```python
from build123d import *

# Parameters (mm, degrees)
EXTRUDE003_DEPTH           = 10
EXTRUDE003_PLACEMENT_ANGLE = 90
SKETCH002_R                = 2.7
EXTRUDE002_DEPTH           = 25
SKETCH001_R                = 5.2
EXTRUDE001_DEPTH           = 6
SKETCH_R                   = 13
SKETCH_R_2                 = 1.65
EXTRUDE_DEPTH              = 5
BOX002_W                   = 43
BOX002_H                   = 42.3
BOX002_DEPTH               = 20
CHAMFER_SIZE               = 4
BOX001_W                   = 20.5
BOX001_H                   = 20.5
BOX001_DEPTH               = 25
BOX_W                      = 63.5
BOX_H                      = 71
BOX_DEPTH                  = 25
CHAMFER001_1_SIZE          = 15
CHAMFER001_2_SIZE          = 2
FILLET_R                   = 1


with BuildPart() as obj1:
    # Sketch003 → Extrude003 (new body)
    with BuildSketch(Plane.YZ):
        with BuildLine():
            ThreePointArc((-3.676943, 3.676968), (0, -5.2), (3.676943, 3.676968))
            Line((2.153911, 5.2), (3.676943, 3.676968))
            Line((-2.153911, 5.2), (2.153911, 5.2))
            Line((-3.676943, 3.676968), (-2.153911, 5.2))
        make_face()
    extrude(amount=EXTRUDE003_DEPTH)


with BuildPart() as obj1_1:
    # Extrude003 placement: moved
    add(obj1.part.moved(Location((42, 62, 10.2))).rotate(Axis((42, 62, 10.2), (0, 0, 1)), EXTRUDE003_PLACEMENT_ANGLE))


with BuildPart() as obj2:
    # Sketch002 → Extrude002 (new body)
    with BuildSketch(Plane.XY):
        with Locations((31.5, 10.25)):
            Circle(SKETCH002_R)
        with Locations((52.5, 10.25)):
            Circle(SKETCH002_R)
        with Locations((10.25, 32.5)):
            Circle(SKETCH002_R)
        with Locations((10.25, 58.8)):
            Circle(SKETCH002_R)
    extrude(amount=EXTRUDE002_DEPTH)


with BuildPart() as huecos:
    # Sketch001 → Extrude001 (new body)
    with BuildSketch(Plane.XY):
        with Locations((31.5, 10.25)):
            Circle(SKETCH001_R)
        with Locations((52.5, 10.25)):
            Circle(SKETCH001_R)
        with Locations((10.25, 32.5)):
            Circle(SKETCH001_R)
        with Locations((10.25, 58.8)):
            Circle(SKETCH001_R)
    extrude(amount=EXTRUDE001_DEPTH)

    # Fusion001: union obj2
    add(obj2.part)

    # Fusion002: union obj1
    add(obj1_1.part)


with BuildPart() as agujero_motor:
    # Sketch → Extrude (new body)
    with BuildSketch(Plane(origin=(20.5, 20.5, 25), x_dir=(1, 0, 0), z_dir=(0, 0, 1))):
        with Locations((21.5, 21.5)):
            Circle(SKETCH_R)
        with Locations((6, 37)):
            Circle(SKETCH_R_2)
        with Locations((37, 37)):
            Circle(SKETCH_R_2)
        with Locations((37, 6)):
            Circle(SKETCH_R_2)
        with Locations((6, 6)):
            Circle(SKETCH_R_2)
    extrude(amount=EXTRUDE_DEPTH)


with BuildPart() as agujero_motor_1:
    # Extrude placement: moved
    add(agujero_motor.part.moved(Location((0, 0, -25))))


with BuildPart() as hueco_motor_total:
    # Box002 → Box002 (new body)
    with BuildSketch(Plane(origin=(20.5, 20.5, 5), x_dir=(1, 0, 0), z_dir=(0, 0, 1))):
        with Locations((21.5, 21.15)):
            Rectangle(BOX002_W, BOX002_H)
    extrude(amount=BOX002_DEPTH)

    # Chamfer
    chamfer_edges = [hueco_motor_total.edges().sort_by_distance(p)[0] for p in [
        (20.5, 20.5, 15),
        (20.5, 62.8, 15),
    ]]
    chamfer(chamfer_edges, length=CHAMFER_SIZE)

    # Fusion: union agujero_motor
    add(agujero_motor_1.part)


with BuildPart() as obj3:
    # Box001 → Box001 (new body)
    with BuildSketch(Plane.XY):
        with Locations((10.25, 10.25)):
            Rectangle(BOX001_W, BOX001_H)
    extrude(amount=BOX001_DEPTH)


with BuildPart() as obj4:
    # Box → Box (new body)
    with BuildSketch(Plane.XY):
        with Locations((31.75, 35.5)):
            Rectangle(BOX_W, BOX_H)
    extrude(amount=BOX_DEPTH)

    # Cut: cut obj3
    add(obj3.part, mode=Mode.SUBTRACT)

    # Cut001: cut hueco_motor_total
    add(hueco_motor_total.part, mode=Mode.SUBTRACT)

    # Cut002: cut huecos
    add(huecos.part, mode=Mode.SUBTRACT)

    # Chamfer001 1
    chamfer001_1_edges = [obj4.edges().sort_by_distance(p)[0] for p in [
        (63.5, 66.9, 25),
    ]]
    chamfer(chamfer001_1_edges, length=CHAMFER001_1_SIZE)

    # Chamfer001 2
    chamfer001_2_edges = [obj4.edges().sort_by_distance(p)[0] for p in [
        (63.5, 10.25, 25),
    ]]
    chamfer(chamfer001_2_edges, length=CHAMFER001_2_SIZE)

    # Fillet
    fillet_edges = [obj4.edges().sort_by_distance(p)[0] for p in [
        (63.5, 71, 5),
        (0, 71, 12.5),
        (0, 20.5, 12.5),
        (20.5, 0, 12.5),
        (63.5, 0, 11.5),
    ]]
    fillet(fillet_edges, radius=FILLET_R)


solid = obj4.part
```
The listing builds one solid part. Answer for the finished solid, in the listing's coordinates (mm). A direction names the side the tool comes from. Give positions to 0.01 mm unless a question says otherwise; leave off trailing zeros. Order: outer loops, then holes, each group sorted by start corner. A loop starts at its lowest first (then second) coordinate and runs counter-clockwise, first axis right, second up. Notation, with made-up numbers: (39.5, -29) -> (60.5, -29) arc R25 ccw to (60.5, 1) -> close; hole circle Ø10 at (45, 89.5). An arc over 180 degrees is marked (long way). Write each question's results on one line, items separated by ' | '.
Q1. The part is cut by section D-D, the plane x = 10.25. Give the vertices of the cut face in (y, z), and give its area (4 significant figures).
Checked values:
outline: (20.5, 0) -> (27.3, 0) -> (27.3, 6) -> (29.8, 6) -> (29.8, 25) -> (20.5, 25) -> close; (35.2, 6) -> (37.7, 6) -> (37.7, 0) -> (53.6, 0) -> (53.6, 6) -> (56.1, 6) -> (56.1, 25) -> (35.2, 25) -> close; (61.5, 6) -> (64, 6) -> (64, 0) -> (71, 0) -> (71, 25) -> (61.5, 25) -> close | area: 932.5 mm^2
Q2. The part is cut by section B-B, the plane z = 3.5. State how many separate pieces and enclosed holes the cut face has, and give its area (3 significant figures).
Checked values:
separate pieces: 1 | enclosed holes: 9 | area: 3,180 mm^2
Q3. The part is cut by section C-C, the plane z = 12. Give the vertices of the cut face in (x, y), and give its area (3 significant figures).
Checked values:
outline: (0, 21.5) arc R1 ccw to (1, 20.5) -> (20.5, 20.5) -> (20.5, 1) arc R1 ccw to (21.5, 0) -> (62.5, 0) arc R1 ccw to (63.5, 1) -> (63.5, 20.5) -> (24.5, 20.5) -> (20.5, 24.5) -> (20.5, 58.8) -> (24.5, 62.8) -> (37.12, 62.8) -> (37.12, 71) -> (1, 71) arc R1 ccw to (0, 70) -> close; (46.88, 62.8) -> (61.5, 62.8) -> (61.5, 71) -> (46.88, 71) -> close; hole circle Ø5.4 at (10.25, 32.5); hole circle Ø5.4 at (10.25, 58.8); hole circle Ø5.4 at (31.5, 10.25); hole circle Ø5.4 at (52.5, 10.25) | area: 2,100 mm^2
Q4. Each of these flat-tipped pins is pushed along its axis until it touches: P1, Ø9.5, axis at x = 52.5, y = 10.25, coming from the -Z side; P2, Ø4, axis at x = 26.5, y = 26.5, coming from the +Z side; P3, Ø6, axis at x = 15.5, z = 6.5, coming from the -Y side. Where does it stop, or does it pass through?
Checked values:
P1: stops at z = 6 | P2: stops at z = 5 | P3: stops at y = 20.5
Q5. The part is cut by section A-A, the plane y = 26.5. Give the vertices of the cut face in (x, z).
Checked values:
outline: (0, 0) -> (24.85, 0) -> (24.85, 5) -> (20.5, 5) -> (20.5, 25) -> (0, 25) -> close; (28.15, 0) -> (55.85, 0) -> (55.85, 5) -> (28.15, 5) -> close; (59.15, 0) -> (63.5, 0) -> (63.5, 5) -> (59.15, 5) -> close
Q6. Determine the mould class of faces 1 (the face through (0, 45, 12)), 2 (the face through (22.5, 60.8, 14.9)), 3 (the face through (25.284, 27.615, 2.465)), 4 (the face through (17, 36, 25)) for opening direction X: pulls with the +X half, pulls with the -X half, needs draft (parallel to the pull), parting line crosses it, or undercut.
Checked values:
face 1: pulls with the -X half | face 2: pulls with the +X half | face 3: undercut | face 4: needs draft
Q7. Which of the six approach directions +Z, -Z, +X, -X, +Y, -Y give full straight-line access (tool end or side, diameter ignored) to faces 5 (the face through (51.3, 51.3, 5)), 6 (the face through (42, 0, 12)), 7 (the face through (20.5, 11, 12)), 8 (the face through (44.926, 66.843, 14.628)), 9 (the face through (12, 30, 6))?
Checked values:
face 5: +Z, +X | face 6: +Z, -Z, +X, -X, -Y | face 7: +Z, -Z, -X, -Y | face 8: +Y | face 9: -Z
Q8. Straight lines are drawn through the part: probe 1 along Y at (x, z) = (10.25, 4.55); probe 2 along X at (y, z) = (10.25, 10.5); probe 3 along Y at (x, z) = (58, 9.5). For each, find the intervals that lie inside material, in ascending order. Write a range as from..to.
Checked values:
probe 1: y = 20.5..27.3, 37.7..53.6, 64..71 | probe 2: x = 20.5..28.8, 34.2..49.8, 55.2..63.5 | probe 3: y = 0..20.5, 62.8..71
